The listing builds one solid part. Answer for the finished solid, in the listing's coordinates (mm). Round coordinates to 2 decimals unless told otherwise and drop trailing zeros. Write each loop counter-clockwise with the first axis right and the second up, starting at its lowest first coordinate (ties: lowest second). Pieces come first, ordered by that corner, then holes. Notation, with made-up numbers: (21.25, 22.25) - (75.25, 22.25) arc R13 ccw to (75.25, 30.25) - close; hole circle Ø5 at (22, 87.25). An arc over 180 degrees is marked (long way). Use a Markdown table: item, result. Add a question column.
1) Each of these flat-tipped pins is pushed along its axis until it touches: P1, Ø4, axis at x = 0, z = -380, coming from the -Y side; P2, Ø4, axis at x = -0.5, z = -200, coming from the +Y side; P3, Ø1, axis at y = 8, z = -219, coming from the -X side. Where does it stop, or does it pass through?
2) A cutting plane is placed at A-A (z = -249). Give the vertices of the cut face in (x, y).
3) Find the intervals of material crossed by probe 1 along X at (y, z) = (12.2, -80); probe 2 along X at (y, z) = (2.25, -80); probe 3 along Y at (x, z) = (6.75, -216), in increasing order. Write a range as from..to.
4) A cutting plane is placed at B-B (x = 0). State how many separate pieces and enclosed holes the cut face has, then the cut area to 3 significant figures.
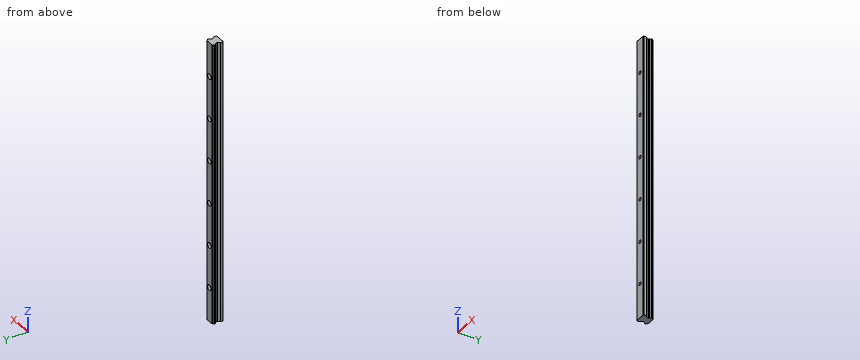
```python
from build123d import *

# Parameters (mm, degrees)
EXTRUDE1_DEPTH     = 460
LPATTERN1_COUNT    = 8
LPATTERN1_PITCH    = 60
SKETCH3_W          = 14.070767507
SKETCH3_H          = 31.75
SKETCH3_W_2        = 7.701339385
SKETCH3_W_3        = 13.600014428
SKETCH3_R          = 2.25
SKETCH3_H_2        = 31.756
CUT_EXTRUDE1_DEPTH = 461.305605006


with BuildPart() as part:
    # Sketch1 → Extrude1 (new body)
    with BuildSketch(Plane(origin=(-20, 0, 0), x_dir=(1, 0, 0), z_dir=(0, 0, 1))):
        with BuildLine():
            Line((12.5, 0.69999271), (13.199992786, 0))
            Line((13.199992786, 0), (26.800007214, 0))
            Line((26.800007214, 0), (27.5, 0.69999271))
            Line((27.5, 0.69999271), (27.5, 4.2000246))
            Line((27.5, 4.2000246), (24.8000183, 6.9000063))
            Line((24.8000183, 6.9000063), (24.8000183, 8.8400054))
            Line((24.8000183, 8.8400054), (25.755946813, 9.794179118))
            ThreePointArc((25.755946813, 9.794179118), (26.198484624, 10.690600567), (27.09432569, 11.13431209))
            Line((27.09432569, 11.13431209), (27.5, 11.5399866))
            Line((27.5, 11.5399866), (27.5, 12.8500204))
            Line((27.5, 12.8500204), (27.09432569, 13.268442751))
            ThreePointArc((27.09432569, 13.268442751), (26.202460867, 13.706434947), (25.755946813, 14.594063938))
            Line((25.755946813, 14.594063938), (25.3500197, 15))
            Line((25.3500197, 15), (14.6499803, 15))
            Line((14.6499803, 15), (14.244053187, 14.594063938))
            ThreePointArc((14.244053187, 14.594063938), (13.797539133, 13.706434947), (12.90567431, 13.268442751))
            Line((12.90567431, 13.268442751), (12.5, 12.8500204))
            Line((12.5, 12.8500204), (12.5, 11.5399866))
            Line((12.5, 11.5399866), (12.90567431, 11.13431209))
            ThreePointArc((12.90567431, 11.13431209), (13.801515376, 10.690600567), (14.244053187, 9.794179118))
            Line((14.244053187, 9.794179118), (15.1999817, 8.8400054))
            Line((15.1999817, 8.8400054), (15.1999817, 6.9000063))
            Line((15.1999817, 6.9000063), (12.5, 4.2000246))
            Line((12.5, 4.2000246), (12.5, 0.69999271))
        make_face()
    extrude(amount=-EXTRUDE1_DEPTH)

    # Sketch2 → Cut-Revolve1 (revolve, cut)
    with BuildSketch(Plane(origin=(0, 0, 0), x_dir=(0, 0, -1), z_dir=(1, 0, 0)), mode=Mode.PRIVATE) as cut_revolve1_sk:
        Polygon((20, 15), (23.75, 15), (23.75, 9.7), (22.25, 9.7), (22.25, 0), (20, 0), align=None)
    cut_revolve1 = revolve(cut_revolve1_sk.sketch.rotate(Axis((0, 0, -20), (0, 1, 0)), 180), axis=Axis((0, 0, -20), (0, 1, 0)), mode=Mode.SUBTRACT)

    # LPattern1: Cut-Revolve1 ×8
    with Locations(*[(0, 0, -i * LPATTERN1_PITCH) for i in range(1, LPATTERN1_COUNT)]):
        add(cut_revolve1, mode=Mode.SUBTRACT)

    # Sketch3 → Cut-Extrude1 (cut, through all)
    # profile 1 of 5: a face of its own
    with BuildSketch(Plane.XZ):
        Polygon((14.501346599, -428.244), (6.800007214, -428.244), (6.800007214, -460), (-6.800007214, -460), (-6.800007214, -428.244), (-9.550443118, -428.244), (-17.163711418, -428.244), (-17.163711418, -476.007491712), (14.501346599, -476.007491712), align=None)
    # profile 2 of 5: a face of its own
    with BuildSketch(Plane.XZ):
        with Locations((-13.835390968, -15.875)):
            Rectangle(SKETCH3_W, SKETCH3_H)
    # profile 3 of 5: a face of its own
    with BuildSketch(Plane.XZ):
        with Locations((10.650676907, -15.875)):
            Rectangle(SKETCH3_W_2, SKETCH3_H)
    # profile 4 of 5: a face of its own
    with BuildSketch(Plane.XZ):
        with Locations((0, -15.875)):
            Rectangle(SKETCH3_W_3, SKETCH3_H)
        with Locations((0, -20)):
            Circle(SKETCH3_R, mode=Mode.SUBTRACT)
    # profile 5 of 5: a face of its own
    with BuildSketch(Plane.XZ):
        with Locations((0, -444.122)):
            Rectangle(SKETCH3_W_3, SKETCH3_H_2)
        with Locations((0, -440)):
            Circle(SKETCH3_R, mode=Mode.SUBTRACT)
    extrude(amount=-CUT_EXTRUDE1_DEPTH, mode=Mode.SUBTRACT)


solid = part.part
```
Entries:
| question | item | result |
|---|---|---|
| 1 | P1 | passes through |
| 1 | P2 | stops at y = 9.7 |
| 1 | P3 | stops at x = -4.8 |
| 2 | outline | (-7.5, 0.7) - (-6.8, 0) - (6.8, 0) - (7.5, 0.7) - (7.5, 4.2) - (4.8, 6.9) - (4.8, 8.84) - (5.76, 9.79) arc R1.56 cw to (7.09, 11.13) - (7.5, 11.54) - (7.5, 12.85) - (7.09, 13.27) arc R1.56 cw to (5.76, 14.59) - (5.35, 15) - (-5.35, 15) - (-5.76, 14.59) arc R1.56 cw to (-7.09, 13.27) - (-7.5, 12.85) - (-7.5, 11.54) - (-7.09, 11.13) arc R1.56 cw to (-5.76, 9.79) - (-4.8, 8.84) - (-4.8, 6.9) - (-7.5, 4.2) - close |
| 3 | probe 1 | x = -7.5..-3.75, 3.75..7.5 |
| 3 | probe 2 | x = -7.5..-2.25, 2.25..7.5 |
| 3 | probe 3 | y = 0..4.95, 11.05..13.36 |
| 4 | separate pieces | 7 |
| 4 | enclosed holes | 0 |
| 4 | area | 5,450 mm² |
